Autodesk Fusion 360 part; units mm, degrees
sketch "Sketch1" plane through (0, 0, 0) normal (0, 0, 1) x (1, 0, 0)
  line L0 (50, -108) -> (50, -39.3754)
  line L1 (50, -39.3754) -> (38.2856, -32.6121)
  spline S0 degree 3 poles (38.2856, -32.6121) (37.4771, -32.1422) (36.6924, -32.1202) (35.8815, -32.5337) (35.0622, -32.9516) (34.2278, -33.9044) (33.6842, -35.2367) (33.2499, -36.3014) (33.0037, -37.5868) (33, -38.8754) knots -0.361367 -0.361367 -0.361367 -0.361367 0.324344 0.324344 0.324344 1.017159 1.017159 1.017159 1.570796 1.570796 1.570796 1.570796
  line L2 (33, -38.8754) -> (33, -125)
  line L3 (33, -125) -> (50, -108)
  line L4 (49.8, -107.9172) -> (49.8, -39.4909)
  line L5 (49.8, -39.4909) -> (38.1854, -32.7852)
  spline S1 degree 3 poles (38.1854, -32.7852) (38.1853, -32.7851) (38.1852, -32.7851) (38.1851, -32.785) (37.4228, -32.342) (36.7342, -32.3234) (35.9723, -32.7119) (35.2137, -33.0988) (34.3985, -34.0153) (33.8694, -35.3123) (33.4463, -36.3493) (33.2036, -37.6124) (33.2, -38.876) knots -0.361437 -0.361437 -0.361437 -0.361437 -0.361367 -0.361367 -0.361367 0.324344 0.324344 0.324344 1.017159 1.017159 1.017159 1.570796 1.570796 1.570796 1.570796
  line L6 (33.2, -38.876) -> (33.2, -124.5172)
  line L7 (33.2, -124.5172) -> (49.8, -107.9172)
  dimension "d1" = 45
  dimension "d2" = 17
  dimension "d3" = 33
  dimension "d4" = 125
  dimension "d5" = 120
  dimension "d6" = 0.5
  dimension "d7" = -0.2
extrude "Extrude1" add sketch "Sketch1" along normal blind 0.6 contours L4 L5 S1 L6 L7
Work out the finished part from the listing and answer in its coordinate system (mm). Give positions to 0.01 mm unless a question says otherwise; leave off trailing zeros. Write each loop counter-clockwise with the first axis right and the second up, starting at its lowest first coordinate (ties: lowest second). Pieces come first, ordered by that corner, then holes. Notation, with made-up numbers: (65.25, -39.5) -> (118.25, -39.5) arc R30 ccw to (118.25, -0.5) -> close; hole circle Ø11 at (2.5, 74.5). An arc over 180 degrees is marked (long way). Write item = value, one per line.
Q1. Consider line 1 along Y through (x, z) = (48.5, 0.3); line 2 along Y through (x, z) = (38.5, 0.25); line 3 along X through (y, z) = (-118.5, 0.25). Determine where each line is inside the solid, lowest interval first.
Computed values:
line_1 = -109.22 to -38.74
line_2 = -119.22 to -32.97
line_3 = 33.2 to 39.22
Q2. Section B-B on y = -112 is taken. Determine the outline of the cut face in (x, z), and give its area (3 significant figures).
Computed values:
outline = (33.2, 0) -> (45.72, 0) -> (45.72, 0.6) -> (33.2, 0.6) -> close
area = 7.51 mm^2
Q3. Section A-A on x = 48.75 is taken. Determine the outline of the cut face in (y, z).
Computed values:
outline = (-108.97, 0) -> (-38.88, 0) -> (-38.88, 0.6) -> (-108.97, 0.6) -> close
